Check sheet for the modelled part. Datum: model origin and axes. Units: mm. Give positions to 0.01 mm unless a question says otherwise; leave off trailing zeros. Loops run counter-clockwise (first coordinate to the right, second up) from the corner with the lowest first, then second, coordinate; pieces in that order, holes last. Notation, with made-up numbers: M 2,7.5 L 59,7.5 A27 cw 59,25.5 Z; hole C -11.75,-2 d7. An arc over 180 degrees is marked long. Use one line per item in the form item = value.
from build123d import *

# Parameters (mm, degrees)
BOSS_EXTRUDE1_DEPTH = 3.2
FILLET1_R           = 2
SKETCH2_R           = 1.6
CUT_EXTRUDE1_DEPTH  = 99.11525581


with BuildPart() as part:
    # Sketch1 → Boss-Extrude1 (new body)
    with BuildSketch(Plane.XY):
        with BuildLine():
            Line((-11.908609546, 96.641044089), (-10.753969279, 88.980506454))
            ThreePointArc((-10.753969279, 88.980506454), (0, 89.628), (10.753969279, 88.980506454))
            Line((10.753969279, 88.980506454), (11.908609546, 96.641044089))
            ThreePointArc((11.908609546, 96.641044089), (0, 97.372), (-11.908609546, 96.641044089))
        make_face()
    extrude(amount=BOSS_EXTRUDE1_DEPTH)

    # Fillet1
    fillet1_edges = [part.edges().sort_by_distance(p)[0] for p in [
        (11.908609546, 96.641044089, 1.6),
        (10.753969279, 88.980506454, 1.6),
        (-10.753969279, 88.980506454, 1.6),
        (-11.908609546, 96.641044089, 1.6),
    ]]
    fillet(fillet1_edges, radius=FILLET1_R)

    # Sketch2 → Cut-Extrude1 (cut, through all)
    with BuildSketch(Plane.XY.offset(3.2)):
        with Locations((-5.670312341, 93.250077468)):
            Circle(SKETCH2_R)
        with Locations((5.670312341, 93.250077468)):
            Circle(SKETCH2_R)
    extrude(amount=-CUT_EXTRUDE1_DEPTH, mode=Mode.SUBTRACT)


solid = part.part
1) Scan lines: line 1 (X direction, y = 92, z = 1.4); line 2 (X direction, y = 92.75, z = 2.95); line 3 (X direction, y = 95, z = 2.75). Record each from-to range of solid material in increasing order.
Evaluation:
line_1 = -11.21 to -6.67, -4.67 to 4.67, 6.67 to 11.21
line_2 = -11.32 to -7.19, -4.15 to 4.15, 7.19 to 11.32
line_3 = -11.62 to 11.62
2) Release check for a two-part mould opening along Y. For faces 1 (the face through (11.316, 92.708, 1.578)), 2 (the face through (0, 93, 0)), 3 (the face through (-5.879, 94.836, 1.622)) record: pulls with the +Y half, pulls with the -Y half, needs draft (parallel to the pull), parting line crosses it, or undercut.
Evaluation:
face_1 = pulls with the -Y half
face_2 = needs draft
face_3 = undercut
3) Section check B-B (x = 4.75). Record the cut outline in (y, z).
Evaluation:
outline = M 89.5,0 L 91.94,0 L 91.94,3.2 L 89.5,3.2 Z; M 94.56,0 L 97.26,0 L 97.26,3.2 L 94.56,3.2 Z
4) Section check A-A (y = 93.5). Record the cut outline in (x, z).
Evaluation:
outline = M -11.44,0 L -7.25,0 L -7.25,3.2 L -11.44,3.2 Z; M -4.09,0 L 4.09,0 L 4.09,3.2 L -4.09,3.2 Z; M 7.25,0 L 11.44,0 L 11.44,3.2 L 7.25,3.2 Z
5) Depth check by flat-ended pin: pin 1 Ø1.5 at (x, z) = (4.5, 0.5) entering from -Y; pin 2 Ø1.9 at (x, y) = (-5.67, 93.25) entering from +Z; pin 3 Ø1 at (x, z) = (4, 0.5) entering from +Y; pin 4 Ø1.5 at (x, z) = (7, 2) entering from +Y. Enter the tip coordinate at first touch or a pass-through.
Evaluation:
pin_1 = 89.47
pin_2 = through
pin_3 = 97.31
pin_4 = 97.17
6) Section check D-D (x = -7). Record the cut outline in (y, z), then the cut area to 3 significant figures.
Evaluation:
outline = M 89.35,0 L 92.36,0 L 92.36,3.2 L 89.35,3.2 Z; M 94.14,0 L 97.12,0 L 97.12,3.2 L 94.14,3.2 Z
area = 19.2 mm^2
7) Section check C-C (z = 2.85). Record the cut outline in (x, y), then the cut area to 3 significant figures.
Evaluation:
outline = M -11.6,94.59 L -11.04,90.88 A2 ccw -8.86,89.19 A89.63 cw 8.86,89.19 A2 ccw 11.04,90.88 L 11.6,94.59 A2 ccw 9.82,96.88 A97.37 ccw -9.82,96.88 A2 ccw Z; hole C -5.67,93.25 d3.2; hole C 5.67,93.25 d3.2
area = 156 mm^2
